```python
from build123d import *

# Parameters (mm, degrees)
F0_R        = 5
F0_R_2      = 3
F1_DEPTH    = 120
F1_FACE_R   = 5
F1_FACE_R_2 = 3


with BuildPart() as f1:
    # F0 (on Right) → F1 (new body)
    with BuildSketch(Plane.YZ):
        Circle(F0_R)
        Circle(F0_R_2, mode=Mode.SUBTRACT)
    extrude(amount=-F1_DEPTH)

    # F3: sweep along a path in F2
    with BuildLine(Plane.XZ) as f3_path:
        ThreePointArc((0, 0), (21.213203, -8.786797), (30, -30))
        Line((30, -30), (30, -60))
    # F1_face (on face) → F3 (sweep)
    with BuildSketch(Plane.YZ):
        Circle(F1_FACE_R)
        Circle(F1_FACE_R_2, mode=Mode.SUBTRACT)
    sweep(path=f3_path.line)


solid = f1.part
```
Part model, mm, in its own coordinate system. Coordinates: 2 decimals unless noted, no trailing zeros. Order: outer loops, then holes, each group sorted by start corner. A loop starts at its lowest first (then second) coordinate and runs counter-clockwise, first axis right, second up. Notation, with made-up numbers: (-15, 74) - (5, 74) arc R22 cw to (5, 89) - close; hole circle Ø8 at (18, 36). An arc over 180 degrees is marked (long way). Return JSON: item names as keys, results as strings. Group by question number.
Item 1: Cut at A-A (x = -65). List the corners of the cut face in (y, z).
Item 2: Pull direction Y, two halves, no side cores. Call faces 1 (the face through (-59, -3, 0)), 2 (the face through (30.1, -3.3, -60)), 3 (the face through (-59.16, -1.08, -4.88)): pulls with the +Y half, pulls with the -Y half, needs draft (parallel to the pull), parting line crosses it, or undercut.
Item 3: Pin check, flat tips, straight feed: pin 1 (6 mm diameter, centred on y = -2, z = -36.5, fed in from +X); pin 2 (1.5 mm diameter, centred on y = -0.5, z = -13.5, fed in from +X); pin 3 (1.5 mm diameter, centred on x = -60, y = 3, fed in from +Z); pin 4 (1 mm diameter, centred on y = 0.5, z = -31, fed in from -X). Stop position of each tip, or through.
Item 4: Drill centre lines: probe 1 along Z at (x, y) = (-57.5, 0); probe 2 along Z at (x, y) = (15.5, 1.75); probe 3 along X at (y, z) = (-0.5, -52). Where is each one in solid material? Low to high. Write a range as from..to.
Check values:
{
 "1": {"outline": "circle Ø10 at (0, 0); hole circle Ø6 at (0, 0)"},
 "2": {"face 1": "undercut", "face 2": "needs draft", "face 3": "parting line crosses it"},
 "3": {"pin 1": "stops at x = 35", "pin 2": "stops at x = 31.23", "pin 3": "stops at z = 4.47", "pin 4": "stops at x = 25"},
 "4": {"probe 1": "z = -5..-3, 3..5", "probe 2": "z = -9.98..-7.21, -1.51..1.03", "probe 3": "x = 25.03..27.04, 32.96..34.97"}
}
